Read the model definition and answer for the solid it produces. Units are mm, in the model's axes. Coordinates: 2 decimals unless noted, no trailing zeros. Order: outer loops, then holes, each group sorted by start corner. A loop starts at its lowest first (then second) coordinate and runs counter-clockwise, first axis right, second up.
```python
from build123d import *

# Parameters (mm, degrees)
SKETCH1_R           = 2.1
SKETCH1_R_2         = 4
SKETCH1_R_3         = 8
BOSS_EXTRUDE1_DEPTH = 5


with BuildPart() as part:
    # Sketch1 → Boss-Extrude1 (new body)
    with BuildSketch(Plane.XY):
        Polygon((124.111470678, 15.338509317), (59.111470678, 15.338509317), (59.111470678, -6.661490683), (59.111470678, -24.661490683), (124.111470678, -24.661490683), (134.111470678, -24.661490683), (134.111470678, -14.661490683), align=None)
        with Locations((64.111470678, 10.338509317)):
            Circle(SKETCH1_R, mode=Mode.SUBTRACT)
        with Locations((119.111470678, 10.338509317)):
            Circle(SKETCH1_R, mode=Mode.SUBTRACT)
        with Locations((64.111470678, 0.338509317)):
            Circle(SKETCH1_R, mode=Mode.SUBTRACT)
        with Locations((119.111470678, 0.338509317)):
            Circle(SKETCH1_R, mode=Mode.SUBTRACT)
        with Locations((123.111470678, -12.661490683)):
            Circle(SKETCH1_R_2, mode=Mode.SUBTRACT)
        with Locations((98.111470678, -12.661490683)):
            Circle(SKETCH1_R_3, mode=Mode.SUBTRACT)
        with Locations((85.611470678, -12.661490683)):
            Circle(SKETCH1_R, mode=Mode.SUBTRACT)
        with Locations((110.611470678, -12.661490683)):
            Circle(SKETCH1_R, mode=Mode.SUBTRACT)
        with Locations(Location((73.111470678, -12.661490683, 0), (0, 0, 180))):
            Circle(SKETCH1_R_2, mode=Mode.SUBTRACT)
    extrude(amount=BOSS_EXTRUDE1_DEPTH)


solid = part.part
```
1) A flat-ended cylindrical pin translates along its axis: pin 1 Ø2.5 at (x, y) = (64.11, 10.34) entering from -Z. Find the tip coordinate at first contact, or state that the pin passes through.
A:
pin 1: passes through
2) A cutting plane is placed at D-D, the plane x = 72.5. Determine the outline of the cut face in (y, z).
A:
outline: (-24.66, 0) - (-16.61, 0) - (-16.61, 5) - (-24.66, 5) - close; (-8.71, 0) - (15.34, 0) - (15.34, 5) - (-8.71, 5) - close
3) A cutting plane is placed at C-C, the plane z = 2.2. State how many separate pieces and enclosed holes the cut face has, and give its area (3 significant figures).
A:
separate pieces: 1
enclosed holes: 9
area: 2,470 mm2
4) A cutting plane is placed at B-B, the plane y = -15.5. Determine the outline of the cut face in (x, z), and give its area (3 significant figures).
A:
outline: (59.11, 0) - (70.29, 0) - (70.29, 5) - (59.11, 5) - close; (75.93, 0) - (90.63, 0) - (90.63, 5) - (75.93, 5) - close; (105.59, 0) - (120.29, 0) - (120.29, 5) - (105.59, 5) - close; (125.93, 0) - (134.11, 0) - (134.11, 5) - (125.93, 5) - close
area: 244 mm2
5) A cutting plane is placed at A-A, the plane x = 91. Determine the outline of the cut face in (y, z).
A:
outline: (-24.66, 0) - (-16.33, 0) - (-16.33, 5) - (-24.66, 5) - close; (-9, 0) - (15.34, 0) - (15.34, 5) - (-9, 5) - close
6) Straight lines are drawn through the part: line 1 (X direction, y = 9, z = 0.75); line 2 (Y direction, x = 124, z = 3.05); line 3 (X direction, y = -12, z = 2.15). For each, find the intervals that lie inside material, in ascending order.
A:
line 1: x = 59.11 to 62.49, 65.73 to 117.49, 120.73 to 126.22
line 2: y = -24.66 to -16.56, -8.76 to 15.34
line 3: x = 59.11 to 69.17, 77.06 to 83.62, 87.6 to 90.14, 106.08 to 108.62, 112.6 to 119.17, 127.06 to 133.22
7) Determine the mould class of faces 1 (the cylindrical face through (108.514, -12.569, 2.465)), 2 (the flat face through (59.111, -4, 2)), 3 (the flat face through (134.111, -20, 2)) for opening direction X: pulls with the +X half, pulls with the -X half, needs draft (parallel to the pull), parting line crosses it, or undercut.
A:
face 1: undercut
face 2: pulls with the -X half
face 3: pulls with the +X half
